The model under review builds one solid part; all positions refer to its coordinate system, in mm. A direction names the side the tool comes from. Coordinates: 2 decimals unless noted, no trailing zeros. Order: outer loops, then holes, each group sorted by start corner. A loop starts at its lowest first (then second) coordinate and runs counter-clockwise, first axis right, second up. Notation, with made-up numbers: (-15.5, -17) -> (28.5, -17) arc R31 ccw to (28.5, 12) -> close; hole circle Ø1 at (-9, 55.5). An arc over 180 degrees is marked (long way). Use CSV: the item, a comma, the result in double quotes. Start each with the question number.
```python
from build123d import *

# Parameters (mm, degrees)
SKETCH1_R           = 8.5
BOSS_EXTRUDE1_DEPTH = 3
CUT_EXTRUDE2_DEPTH  = 2
BOSS_EXTRUDE4_DEPTH = 6


with BuildPart() as part:
    # Sketch1 → Boss-Extrude1 (new body)
    with BuildSketch(Plane.XY):
        Circle(SKETCH1_R)
    extrude(amount=BOSS_EXTRUDE1_DEPTH)

    # Sketch4 → Cut-Extrude2 (cut)
    with BuildSketch(Plane(origin=(0, 0, 0), x_dir=(-1, 0, 0), z_dir=(0, 0, -1))):
        with BuildLine():
            Line((-3.25, 0.968245837), (3.25, 0.968245837))
            ThreePointArc((3.25, 0.968245837), (7, 0), (3.25, -0.968245837))
            Line((3.25, -0.968245837), (-3.25, -0.968245837))
            ThreePointArc((-3.25, -0.968245837), (-7, 0), (-3.25, 0.968245837))
        make_face()
    extrude(amount=-CUT_EXTRUDE2_DEPTH, mode=Mode.SUBTRACT)

    # Sketch2 → Boss-Extrude4 (add)
    with BuildSketch(Plane.XY.offset(3)):
        with BuildLine():
            Line((3.222464246, 6.910596876), (2.747018701, 5.891000616))
            ThreePointArc((2.747018701, 5.891000616), (1.682323793, 6.278517871), (0.566512328, 6.475265538))
            Line((0.566512328, 6.475265538), (0.664562538, 7.595984573))
            Line((0.664562538, 7.595984573), (0.332281269, 7.985492286))
            Line((0.332281269, 7.985492286), (-0.332281269, 7.985492286))
            Line((-0.332281269, 7.985492286), (-0.664562538, 7.595984573))
            Line((-0.664562538, 7.595984573), (-0.566512328, 6.475265538))
            ThreePointArc((-0.566512328, 6.475265538), (-1.682323793, 6.278517871), (-2.747018701, 5.891000616))
            Line((-2.747018701, 5.891000616), (-3.222464246, 6.910596876))
            Line((-3.222464246, 6.910596876), (-3.704982123, 7.081779816))
            Line((-3.704982123, 7.081779816), (-4.280510164, 6.749498547))
            Line((-4.280510164, 6.749498547), (-4.373520327, 6.246034338))
            Line((-4.373520327, 6.246034338), (-3.728246836, 5.324488288))
            ThreePointArc((-3.728246836, 5.324488288), (-4.596194078, 4.596194078), (-5.324488288, 3.728246836))
            Line((-5.324488288, 3.728246836), (-6.246034338, 4.373520327))
            Line((-6.246034338, 4.373520327), (-6.749498547, 4.280510164))
            Line((-6.749498547, 4.280510164), (-7.081779816, 3.704982123))
            Line((-7.081779816, 3.704982123), (-6.910596876, 3.222464246))
            Line((-6.910596876, 3.222464246), (-5.891000616, 2.747018701))
            ThreePointArc((-5.891000616, 2.747018701), (-6.278517871, 1.682323793), (-6.475265538, 0.566512328))
            Line((-6.475265538, 0.566512328), (-7.595984573, 0.664562538))
            Line((-7.595984573, 0.664562538), (-7.985492286, 0.332281269))
            Line((-7.985492286, 0.332281269), (-7.985492286, -0.332281269))
            Line((-7.985492286, -0.332281269), (-7.595984573, -0.664562538))
            Line((-7.595984573, -0.664562538), (-6.475265538, -0.566512328))
            ThreePointArc((-6.475265538, -0.566512328), (-6.278517871, -1.682323793), (-5.891000616, -2.747018701))
            Line((-5.891000616, -2.747018701), (-6.910596876, -3.222464246))
            Line((-6.910596876, -3.222464246), (-7.081779816, -3.704982123))
            Line((-7.081779816, -3.704982123), (-6.749498547, -4.280510164))
            Line((-6.749498547, -4.280510164), (-6.246034338, -4.373520327))
            Line((-6.246034338, -4.373520327), (-5.324488288, -3.728246836))
            ThreePointArc((-5.324488288, -3.728246836), (-4.596194078, -4.596194078), (-3.728246836, -5.324488288))
            Line((-3.728246836, -5.324488288), (-4.373520327, -6.246034338))
            Line((-4.373520327, -6.246034338), (-4.280510164, -6.749498547))
            Line((-4.280510164, -6.749498547), (-3.704982123, -7.081779816))
            Line((-3.704982123, -7.081779816), (-3.222464246, -6.910596876))
            Line((-3.222464246, -6.910596876), (-2.747018701, -5.891000616))
            ThreePointArc((-2.747018701, -5.891000616), (-1.682323793, -6.278517871), (-0.566512328, -6.475265538))
            Line((-0.566512328, -6.475265538), (-0.664562538, -7.595984573))
            Line((-0.664562538, -7.595984573), (-0.332281269, -7.985492286))
            Line((-0.332281269, -7.985492286), (0.332281269, -7.985492286))
            Line((0.332281269, -7.985492286), (0.664562538, -7.595984573))
            Line((0.664562538, -7.595984573), (0.566512328, -6.475265538))
            ThreePointArc((0.566512328, -6.475265538), (1.682323793, -6.278517871), (2.747018701, -5.891000616))
            Line((2.747018701, -5.891000616), (3.222464246, -6.910596876))
            Line((3.222464246, -6.910596876), (3.704982123, -7.081779816))
            Line((3.704982123, -7.081779816), (4.280510164, -6.749498547))
            Line((4.280510164, -6.749498547), (4.373520327, -6.246034338))
            Line((4.373520327, -6.246034338), (3.728246836, -5.324488288))
            ThreePointArc((3.728246836, -5.324488288), (4.596194078, -4.596194078), (5.324488288, -3.728246836))
            Line((5.324488288, -3.728246836), (6.246034338, -4.373520327))
            Line((6.246034338, -4.373520327), (6.749498547, -4.280510164))
            Line((6.749498547, -4.280510164), (7.081779816, -3.704982123))
            Line((7.081779816, -3.704982123), (6.910596876, -3.222464246))
            Line((6.910596876, -3.222464246), (5.891000616, -2.747018701))
            ThreePointArc((5.891000616, -2.747018701), (6.278517871, -1.682323793), (6.475265538, -0.566512328))
            Line((6.475265538, -0.566512328), (7.595984573, -0.664562538))
            Line((7.595984573, -0.664562538), (7.985492286, -0.332281269))
            Line((7.985492286, -0.332281269), (7.985492286, 0.332281269))
            Line((7.985492286, 0.332281269), (7.595984573, 0.664562538))
            Line((7.595984573, 0.664562538), (6.475265538, 0.566512328))
            ThreePointArc((6.475265538, 0.566512328), (6.278517871, 1.682323793), (5.891000616, 2.747018701))
            Line((5.891000616, 2.747018701), (6.910596876, 3.222464246))
            Line((6.910596876, 3.222464246), (7.081779816, 3.704982123))
            Line((7.081779816, 3.704982123), (6.749498547, 4.280510164))
            Line((6.749498547, 4.280510164), (6.246034338, 4.373520327))
            Line((6.246034338, 4.373520327), (5.324488288, 3.728246836))
            ThreePointArc((5.324488288, 3.728246836), (4.596194078, 4.596194078), (3.728246836, 5.324488288))
            Line((3.728246836, 5.324488288), (4.373520327, 6.246034338))
            Line((4.373520327, 6.246034338), (4.280510164, 6.749498547))
            Line((4.280510164, 6.749498547), (3.704982123, 7.081779816))
            Line((3.704982123, 7.081779816), (3.222464246, 6.910596876))
        make_face()
    extrude(amount=BOSS_EXTRUDE4_DEPTH)


solid = part.part
```
Q1. Clearance check with flat-ended pins moving along their axes: pin 1 Ø0.7 at (x, z) = (0, 6.5) entering from +Y; pin 2 Ø0.5 at (y, z) = (0, 6.5) entering from -X; pin 3 Ø5 at (x, z) = (-5, 4.5) entering from -Y. State where each tip first meets the part, or that it passes through.
Q2. For faces 1 (the flat face through (-5.779, 4.046, 5.958)), 2 (the flat face through (-6.41, 2.99, 5.96)), 3 (the cylindrical face through (4.61, 4.58, 5.96)), 4 (the flat face through (0, 0.968, 1)), 5 (the flat face through (2.98, -6.39, 5.96)), list the 3-axis set-ups (+Z, -Z, +X, -X, +Y, -Y) from which the entire face can be reached by the end or side of a thin tool; tool diameter is ignored.
Q3. Draft analysis for pull direction X (two halves, no side actions). For faces 6 (the flat face through (6.39, 2.98, 5.96)), 7 (the flat face through (0, -0.968, 1)), 8 (the flat face through (0, 0, 9)), state which applies: +X half, -X half, draft (parallel to the pull), parting line (faces both ways), or undercut.
Q4. Add section D-D, the plane y = 3. State the section outline as (x, z) points.
Q5. To check wall thickness, follow probe 1 along Y at (x, z) = (5, 1.2); probe 2 along Z at (x, y) = (3.25, 7); probe 3 along Z at (x, y) = (3.5, 1.25). State the ranges of each line that lie inside material, in increasing order.
Q6. Add section C-C, the plane z = 2.75. State the section outline as (x, y) points.
Q7. Add section A-A, the plane x = 0. State the section outline as (y, z) points, then the cut area to 3 significant figures.
Q8. Add section B-B, the plane y = 0. State the section outline as (x, z) points, then the cut area to 3 significant figures.
Answer block:
1,pin 1,"stops at y = 7.99"
1,pin 2,"stops at x = -7.99"
1,pin 3,"stops at y = -7.95"
2,face 1,"+Z, +Y"
2,face 2,"+Z, -X"
2,face 3,"+Z"
2,face 4,"-Z"
2,face 5,"+Z, -Y"
3,face 6,"+X half"
3,face 7,"undercut"
3,face 8,"draft"
4,outline,"(-7.95, 0) -> (7.95, 0) -> (7.95, 3) -> (6.43, 3) -> (6.43, 9) -> (-6.43, 9) -> (-6.43, 3) -> (-7.95, 3) -> close"
5,probe 1,"y = -6.87 to -2, 2 to 6.87"
5,probe 2,"z = 0 to 3"
5,probe 3,"z = 2 to 9"
6,outline,"circle Ø17 at (0, 0)"
7,outline,"(-8.5, 0) -> (-0.97, 0) -> (-0.97, 2) -> (0.97, 2) -> (0.97, 0) -> (8.5, 0) -> (8.5, 3) -> (7.99, 3) -> (7.99, 9) -> (-7.99, 9) -> (-7.99, 3) -> (-8.5, 3) -> close"
7,area,"143 mm²"
8,outline,"(-8.5, 0) -> (-7, 0) -> (-7, 2) -> (7, 2) -> (7, 0) -> (8.5, 0) -> (8.5, 3) -> (7.99, 3) -> (7.99, 9) -> (-7.99, 9) -> (-7.99, 3) -> (-8.5, 3) -> close"
8,area,"119 mm²"
